Source: CAD feature listing. Evaluate the final solid. Frame: model axes, mm. Face numbers are marked on the shaded views. Give positions to 0.01 mm unless a question says otherwise; leave off trailing zeros. Loops run counter-clockwise (first coordinate to the right, second up) from the corner with the lowest first, then second, coordinate; pieces in that order, holes last. Notation, with made-up numbers: M 30,27.5 L 42,27.5 A33 ccw 42,63.5 Z; hole C 27,25 d6. An arc over 180 degrees is marked long. Answer in a Markdown table with one row per item.
```python
from build123d import *

# Parameters (mm, degrees)
F1_DEPTH = 14.986


with BuildPart() as f1:
    # F0 (on Top) → F1 (new body)
    with BuildSketch(Plane.XY):
        Polygon((57.917436, -24.592009), (-37.311969, 59.433942), (-53.098663, 44.156493), (-20.332476, 15.398937), (-4.358985, 1.37965), (14.88192, -15.507314), (30.111295, -28.87352), (35.677184, -33.758476), (42.639993, -39.869452), (57.917436, -39.869452), align=None)
        Polygon((-4.358985, 1.37965), (-20.332476, 15.398937), (-73.468593, 15.398937), (-73.97784, 1.37965), align=None)
    extrude(amount=F1_DEPTH)


solid = f1.part
```
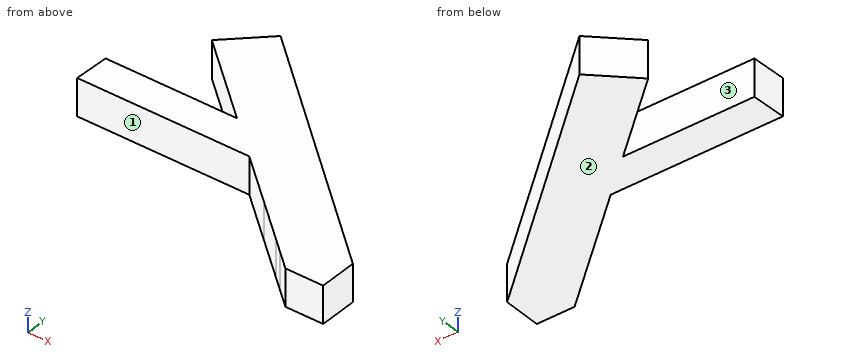
1) Section D-D, the plane x = -54.5. Return loops of the section in (y, z), then the cut area to 3 significant figures.
Reply:
| item | result |
|---|---|
| outline | M 1.38,0 L 15.4,0 L 15.4,14.99 L 1.38,14.99 Z |
| area | 210 mm² |
2) Pin query (flat end, axial travel): pin 1 Ø1.5 at (x, z) = (-51, 6) entering from +Y; pin 2 Ø1.5 at (x, z) = (3.5, 8) entering from -Y; pin 3 Ø4 at (y, z) = (35, 4) entering from -X. Return the tip coordinate at first contact, or that it passes through.
Reply:
| item | result |
|---|---|
| pin 1 | stops at y = 46.91 |
| pin 2 | stops at y = -6.18 |
| pin 3 | stops at x = -44.94 |
3) Section A-A, the plane z = 12. Return loops of the section in (x, y), then the cut area to 3 significant figures.
Reply:
| item | result |
|---|---|
| outline | M -73.98,1.38 L -4.36,1.38 L 42.64,-39.87 L 57.92,-39.87 L 57.92,-24.59 L -37.31,59.43 L -53.1,44.16 L -20.33,15.4 L -73.47,15.4 Z |
| area | 3,740 mm² |
4) Section C-C, the plane y = 32.5. Return loops of the section in (x, z).
Reply:
| item | result |
|---|---|
| outline | M -39.82,0 L -6.79,0 L -6.79,14.99 L -39.82,14.99 Z |
5) Material intervals for L1, parallel to Y at x = -54, z = 10.25; L2, parallel to Y at x = -26, z = 2.75; L3, parallel to Y at x = -53, z = 11.75, sorted ascending.
Reply:
| item | result |
|---|---|
| L1 | y = 1.38 to 15.4 |
| L2 | y = 1.38 to 15.4, 20.37 to 49.45 |
| L3 | y = 1.38 to 15.4, 44.07 to 44.25 |
6) Pull-direction query (Y, two-part tool) for the marked faces 1, 2 and 3; classes: released by +Y, released by -Y, zero draft, split by the parting line, or undercut.
Reply:
| item | result |
|---|---|
| face 1 | released by -Y |
| face 2 | zero draft |
| face 3 | undercut |
7) Section B-B, the plane x = -41. Return loops of the section in (y, z).
Reply:
| item | result |
|---|---|
| outline | M 1.38,0 L 15.4,0 L 15.4,14.99 L 1.38,14.99 Z; M 33.54,0 L 55.86,0 L 55.86,14.99 L 33.54,14.99 Z |
